Read the model definition and answer for the solid it produces. Units are mm, in the model's axes. Coordinates: 2 decimals unless noted, no trailing zeros. Order: outer loops, then holes, each group sorted by start corner. A loop starts at its lowest first (then second) coordinate and runs counter-clockwise, first axis right, second up.
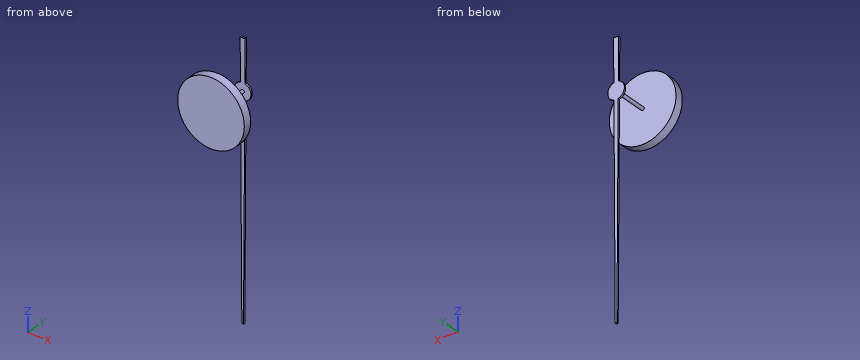
```python
from build123d import *

# Parameters (mm, degrees)
BOSS_EXTRUDE1_DEPTH = 0.1
SKETCH2_R           = 0.1
BOSS_EXTRUDE2_DEPTH = 2
SKETCH3_R           = 2
BOSS_EXTRUDE3_DEPTH = 0.5


with BuildPart() as part:
    # Sketch1 → Boss-Extrude1 (new body)
    with BuildSketch(Plane(origin=(0, 0, 0), x_dir=(1, 0, 0), z_dir=(0, 1, 0))):
        with BuildLine():
            Line((-0.128229515, 0.483277551), (-0.05, 13))
            Line((-0.05, 13), (0.05, 13))
            Line((0.05, 13), (0.128229515, 0.483277551))
            ThreePointArc((0.128229515, 0.483277551), (0.499990235, 0.003124939), (0.134260231, -0.48163699))
            Line((0.134260231, -0.48163699), (0.15, -3))
            Line((0.15, -3), (-0.15, -3))
            Line((-0.15, -3), (-0.134260231, -0.48163699))
            ThreePointArc((-0.134260231, -0.48163699), (-0.499990235, 0.003124939), (-0.128229515, 0.483277551))
        make_face()
    extrude(amount=BOSS_EXTRUDE1_DEPTH)

    # Sketch2 → Boss-Extrude2 (add)
    with BuildSketch(Plane.XZ):
        Circle(SKETCH2_R)
    extrude(amount=BOSS_EXTRUDE2_DEPTH)

    # Sketch3 → Boss-Extrude3 (add)
    with BuildSketch(Plane.XZ.offset(2)):
        Circle(SKETCH3_R)
    extrude(amount=BOSS_EXTRUDE3_DEPTH)


solid = part.part
```
1) A flat-ended cylindrical pin translates along its axis: pin 1 Ø0.5 at (x, z) = (0, -7.5) entering from -Y. Find the tip coordinate at first contact, or state that the pin passes through.
A:
pin 1: stops at y = 0
2) A cutting plane is placed at A-A, the plane z = -1.25. Determine the outline of the cut face in (x, y).
A:
outline: (-1.56, -2.5) - (1.56, -2.5) - (1.56, -2) - (-1.56, -2) - close; (-0.12, 0) - (0.12, 0) - (0.12, 0.1) - (-0.12, 0.1) - close
3) A cutting plane is placed at C-C, the plane z = -5. Determine the outline of the cut face in (x, y), and give its area (3 significant figures).
A:
outline: (-0.1, 0) - (0.1, 0) - (0.1, 0.1) - (-0.1, 0.1) - close
area: 0.0200 mm2
4) A cutting plane is placed at B-B, the plane y = -1.8. Determine the outline of the cut face in (x, z), and give its area (3 significant figures).
A:
outline: circle Ø0.2 at (0, 0)
area: 0.0314 mm2
5) A cutting plane is placed at D-D, the plane x = -0.75. Determine the outline of the cut face in (y, z), and give its area (3 significant figures).
A:
outline: (-2.5, -1.85) - (-2, -1.85) - (-2, 1.85) - (-2.5, 1.85) - close
area: 1.85 mm2
6) A straight line is drawn through the part: line 1 (Y direction, x = 1.5, z = 1.25). Find the intervals that lie inside material, in ascending order.
A:
line 1: y = -2.5 to -2
